Check sheet for the modelled part. Datum: model origin and axes. Units: mm. Face numbers are marked on the shaded views. Round coordinates to 2 decimals unless told otherwise and drop trailing zeros. Order: outer loops, then holes, each group sorted by start corner. A loop starts at its lowest first (then second) coordinate and runs counter-clockwise, first axis right, second up.
```python
from build123d import *

# Parameters (mm, degrees)
SKETCH_1_W          = 394
SKETCH_1_H          = 200
EXTRUDE_1_DEPTH     = 13
SKETCH_2_W          = 394
SKETCH_2_H          = 5
CUT_EXTRUDE_1_DEPTH = 5
CUT_EXTRUDE_2_DEPTH = 363.900192956
CUT_EXTRUDE_3_DEPTH = 8


with BuildPart() as part:
    # ｽｹｯﾁ1 → ﾎﾞｽ - 押し出し1 (new body)
    with BuildSketch(Plane.XY):
        with Locations((127.719868277, 61.507142857)):
            Rectangle(SKETCH_1_W, SKETCH_1_H)
    extrude(amount=EXTRUDE_1_DEPTH)

    # ｽｹｯﾁ2 → ｶｯﾄ - 押し出し1 (cut)
    with BuildSketch(Plane.XY.offset(13)):
        with Locations((127.719868277, -30.992857143)):
            Rectangle(SKETCH_2_W, SKETCH_2_H)
    extrude(amount=-CUT_EXTRUDE_1_DEPTH, mode=Mode.SUBTRACT)

    # ｽｹｯﾁ3 → ｶｯﾄ - 押し出し2 (cut, through all)
    with BuildSketch(Plane.XY.offset(13)):
        with BuildLine():
            Line((27.719868277, 74.007142857), (215.219868277, 74.007142857))
            Line((215.219868277, 74.007142857), (215.219868277, 131.507142857))
            ThreePointArc((215.219868277, 131.507142857), (227.719868277, 144.007142857), (240.219868277, 131.507142857))
            Line((240.219868277, 131.507142857), (240.219868277, -8.492857143))
            ThreePointArc((240.219868277, -8.492857143), (227.719868277, -20.992857143), (215.219868277, -8.492857143))
            Line((215.219868277, -8.492857143), (215.219868277, 49.007142857))
            Line((215.219868277, 49.007142857), (27.719868277, 49.007142857))
            ThreePointArc((27.719868277, 49.007142857), (15.219868277, 61.507142857), (27.719868277, 74.007142857))
        make_face()
    extrude(amount=-CUT_EXTRUDE_2_DEPTH, mode=Mode.SUBTRACT)

    # ｽｹｯﾁ6 → ｶｯﾄ - 押し出し3 (cut)
    with BuildSketch(Plane.XY.offset(13)):
        with BuildLine():
            Line((27.719868277, 84.007142857), (205.219868277, 84.007142857))
            Line((205.219868277, 84.007142857), (205.219868277, 121.507142857))
            ThreePointArc((205.219868277, 121.507142857), (227.719868277, 144.007142857), (250.219868277, 121.507142857))
            Line((250.219868277, 121.507142857), (250.219868277, 84.007142857))
            Line((250.219868277, 84.007142857), (260.219868277, 84.007142857))
            ThreePointArc((260.219868277, 84.007142857), (282.719868277, 61.507142857), (260.219868277, 39.007142857))
            Line((260.219868277, 39.007142857), (250.219868277, 39.007142857))
            Line((250.219868277, 39.007142857), (250.219868277, 1.507142857))
            ThreePointArc((250.219868277, 1.507142857), (227.719868277, -20.992857143), (205.219868277, 1.507142857))
            Line((205.219868277, 1.507142857), (205.219868277, 39.007142857))
            Line((205.219868277, 39.007142857), (27.719868277, 39.007142857))
            ThreePointArc((27.719868277, 39.007142857), (5.219868277, 61.507142857), (27.719868277, 84.007142857))
        make_face()
    extrude(amount=-CUT_EXTRUDE_3_DEPTH, mode=Mode.SUBTRACT)


solid = part.part
```
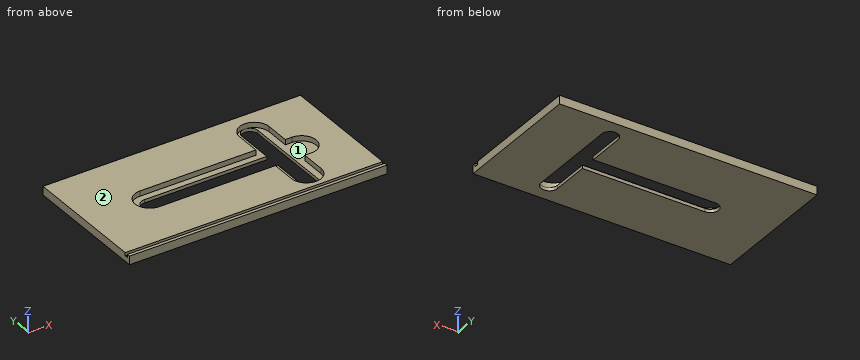
Item 1: Sectioned sample at D-D (y = 45). Record the cut outline in (x, z).
Answer:
outline: (-69.28, 0) - (215.22, 0) - (215.22, 5) - (12.43, 5) - (12.43, 13) - (-69.28, 13) - close; (240.22, 0) - (324.72, 0) - (324.72, 13) - (275.51, 13) - (275.51, 5) - (240.22, 5) - close
Item 2: Scan lines: line 1 along Y through (x, z) = (203.5, 11); line 2 along X through (y, z) = (14, 6.75); line 3 along Y through (x, z) = (123, 3.25). Record each from-to range of solid material in increasing order.
Answer:
line 1: y = -38.49 to -33.49, -28.49 to 39.01, 84.01 to 161.51
line 2: x = -69.28 to 205.22, 250.22 to 324.72
line 3: y = -38.49 to 49.01, 74.01 to 161.51
Item 3: Sectioned sample at B-B (x = 171). Record the cut outline in (y, z).
Answer:
outline: (-38.49, 0) - (49.01, 0) - (49.01, 5) - (39.01, 5) - (39.01, 13) - (-28.49, 13) - (-28.49, 8) - (-33.49, 8) - (-33.49, 13) - (-38.49, 13) - close; (74.01, 0) - (161.51, 0) - (161.51, 13) - (84.01, 13) - (84.01, 5) - (74.01, 5) - close
Item 4: Sectioned sample at C-C (y = 97). Record the cut outline in (x, z).
Answer:
outline: (-69.28, 0) - (215.22, 0) - (215.22, 5) - (205.22, 5) - (205.22, 13) - (-69.28, 13) - close; (240.22, 0) - (324.72, 0) - (324.72, 13) - (250.22, 13) - (250.22, 5) - (240.22, 5) - close
Item 5: Sectioned sample at A-A (z = 10.25). Record the cut outline in (x, y), and give its area (3 significant figures).
Answer:
outline: (-69.28, -38.49) - (324.72, -38.49) - (324.72, -33.49) - (-69.28, -33.49) - close; (-69.28, -28.49) - (324.72, -28.49) - (324.72, 161.51) - (-69.28, 161.51) - close; hole (27.72, 39.01) - (205.22, 39.01) - (205.22, 1.51) arc R22.5 ccw to (250.22, 1.51) - (250.22, 39.01) - (260.22, 39.01) arc R22.5 ccw to (260.22, 84.01) - (250.22, 84.01) - (250.22, 121.51) arc R22.5 ccw to (205.22, 121.51) - (205.22, 84.01) - (27.72, 84.01) arc R22.5 ccw to start
area: 59,800 mm2
Item 6: Release check for a two-part mould opening along X. For the marked faces 1 and 2 record: released by +X, released by -X, zero draft, split by the parting line, or undercut.
Answer:
face 1: undercut
face 2: zero draft
Item 7: Go/stop test with a flat-tipped pin: P1, Ø1.5, axis at x = 226, y = -30, coming from the +Z side. Record where the tip stops, or that it passes through.
Answer:
P1: stops at z = 8
